Verification items for the finished model (mm, model axes). Give positions to 0.01 mm unless a question says otherwise; leave off trailing zeros. Put each result on its own line as item: value.
from build123d import *

# Parameters (mm, degrees)
F_2020_SKETCH_R     = 3
BOSS_EXTRUDE1_DEPTH = 400


with BuildPart() as part:
    # 2020 sketch → Boss-Extrude1 (new body)
    with BuildSketch(Plane(origin=(0, 0, 0), x_dir=(1, 0, 0), z_dir=(0, 1, 0))):
        Polygon((-4, 10), (-4, 8), (-7, 8), (-3, 4), (3, 4), (7, 8), (4, 8), (4, 10), (10, 10), (10, 4), (8, 4), (8, 7), (4, 3), (4, -3), (8, -7), (8, -4), (10, -4), (10, -10), (4, -10), (4, -8), (7, -8), (3, -4), (-3, -4), (-7, -8), (-4, -8), (-4, -10), (-10, -10), (-10, -4), (-8, -4), (-8, -7), (-4, -3), (-4, 3), (-8, 7), (-8, 4), (-10, 4), (-10, 10), align=None)
        with Locations(Location((0, 0, 0), (0, 0, 270))):
            Circle(F_2020_SKETCH_R, mode=Mode.SUBTRACT)
    boss_extrude1 = extrude(amount=BOSS_EXTRUDE1_DEPTH)

    # Mirror1: Boss-Extrude1 across plane
    add(boss_extrude1.mirror(Plane(origin=(10, 400, 4), x_dir=(0, 0, 1), z_dir=(1, 0, 0))))


solid = part.part
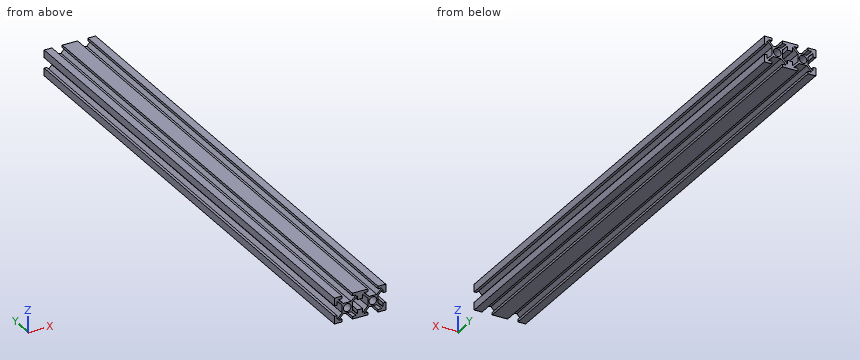
Q1. Scan lines: line 1 along X through (y, z) = (194, 0); line 2 along X through (y, z) = (172, 8.5); line 3 along Z through (x, y) = (20, 111). Record each from-to range of solid material in increasing order.
Answers follow:
line 1: x = -4 to -3, 3 to 4, 16 to 17, 23 to 24
line 2: x = -10 to -4, 4 to 16, 24 to 30
line 3: z = -4 to -3, 3 to 4
Q2. Section check A-A, the plane y = 106. Give the number of separate pieces and of enclosed holes in the cut face, plus the area to 3 significant figures.
Answers follow:
separate pieces: 1
enclosed holes: 3
area: 295 mm2
Q3. Go/stop test with a flat-tipped pin: pin 1 Ø3 at (y, z) = (172.5, 0.5) entering from +X. Record where the tip stops, or that it passes through.
Answers follow:
pin 1: stops at x = 24
